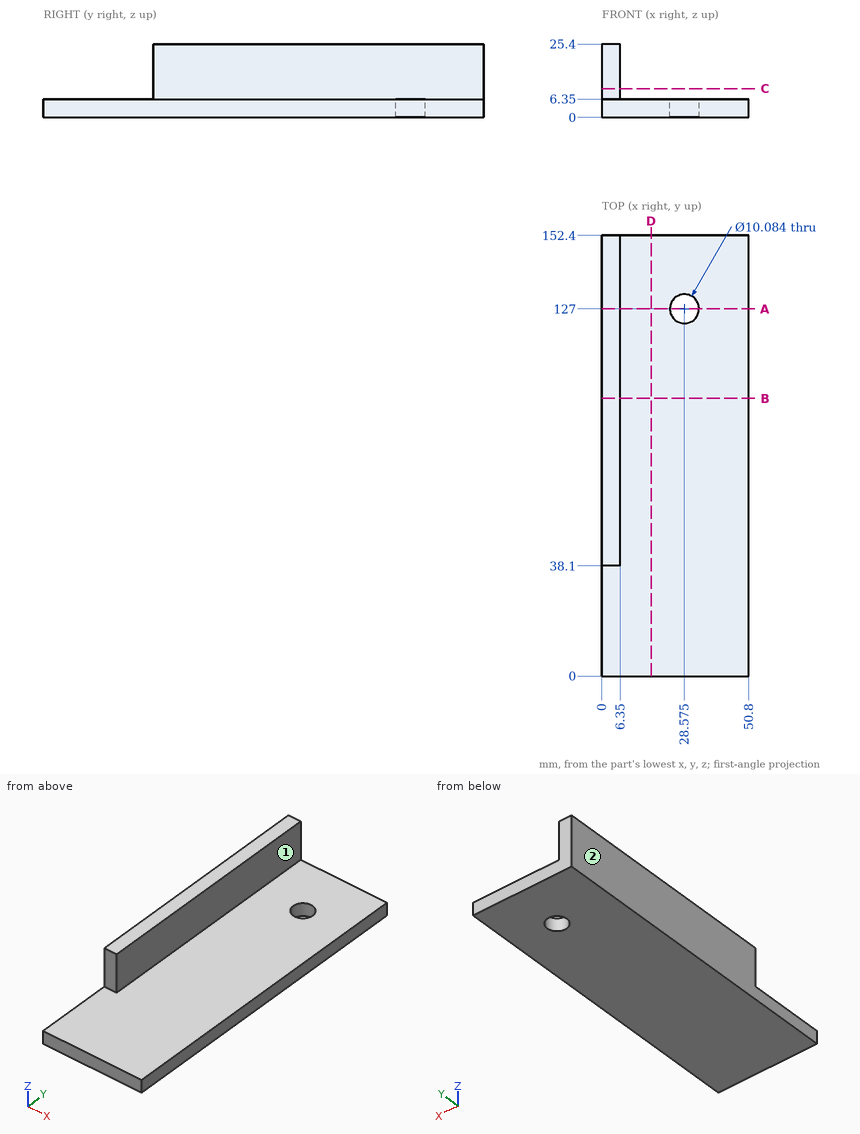
Check sheet for the drawn part. Datum: minimum x, y, z corner. Units: mm. A direction names the side the tool comes from. Round coordinates to 2 decimals unless told otherwise and drop trailing zeros. Order: outer loops, then holes, each group sorted by start corner. A loop starts at its lowest first (then second) coordinate and runs counter-clockwise, first axis right, second up. Notation, with made-up numbers: (53, 66.25) - (85, 66.25) arc R32 cw to (85, 102.25) - close; hole circle Ø7 at (-33, 40). An arc over 180 degrees is marked (long way). Use a Markdown table: item, result. Add a question column.
(1) Sectioned sample at B-B, the plane y = 96. Enter the section's corners in (x, z).
(2) Sectioned sample at C-C, the plane z = 10. Enter the section's corners in (x, y), and give its area (3 significant figures).
(3) Material ranges on line 1 along X through (y, z) = (127, 3); line 2 along Z through (x, y) = (43, 16); line 3 along Y through (x, z) = (4.5, 9.5), recorded low to high. Write a range as [from, to].
(4) Sectioned sample at A-A, the plane y = 127. Enter the section's corners in (x, z).
(5) Sectioned sample at D-D, the plane x = 17. Enter the section's corners in (y, z), and give its area (3 significant figures).
(6) Tool access check on the marked faces 1 and 2. Record the directions out of +Z, -Z, +X, -X, +Y, -Y that give a thin tool (end or side, any length) a straight path to the whole face; none if there is none.
(7) Depth check by flat-ended pin: pin 1 (5 mm diameter, centred on x = 40, y = 130, fed in from +Z); pin 2 (15 mm diameter, centred on y = 111, z = 15, fed in from +X); pin 3 (7 mm diameter, centred on x = 2, z = 19, fed in from -Y). Enter the tip coordinate at first touch or a pass-through.
Answers below:
| question | item | result |
|---|---|---|
| 1 | outline | (0, 0) - (50.8, 0) - (50.8, 6.35) - (6.35, 6.35) - (6.35, 25.4) - (0, 25.4) - close |
| 2 | outline | (0, 38.1) - (6.35, 38.1) - (6.35, 152.4) - (0, 152.4) - close |
| 2 | area | 726 mm² |
| 3 | line 1 | [0, 23.53], [33.62, 50.8] |
| 3 | line 2 | [0, 6.35] |
| 3 | line 3 | [38.1, 152.4] |
| 4 | outline | (0, 0) - (23.53, 0) - (23.53, 6.35) - (6.35, 6.35) - (6.35, 25.4) - (0, 25.4) - close; (33.62, 0) - (50.8, 0) - (50.8, 6.35) - (33.62, 6.35) - close |
| 5 | outline | (0, 0) - (152.4, 0) - (152.4, 6.35) - (0, 6.35) - close |
| 5 | area | 968 mm² |
| 6 | face 1 | +Z, +X, +Y, -Y |
| 6 | face 2 | +Z, -Z, -X, +Y, -Y |
| 7 | pin 1 | z = 6.35 |
| 7 | pin 2 | x = 6.35 |
| 7 | pin 3 | y = 38.1 |
